Could you check a few things on this drawing? It's one solid part, dimensions in mm from its lowest x, y, z. A direction names the side the tool comes from. Give positions to 0.01 mm unless a question says otherwise; leave off trailing zeros. Write each loop counter-clockwise with the first axis right and the second up, starting at its lowest first coordinate (ties: lowest second). Pieces come first, ordered by that corner, then holes. Notation, with made-up numbers: (35, -30) -> (51, -30) arc R31 cw to (51, 3) -> close; hole circle Ø6 at (87.5, 31). An arc over 180 degrees is marked (long way). Answer as CSV lines item,"result". Start each with the question number.
1. If we section it at A-A on y = 29: Write out the boundary of the cut face in (x, z), plus the area to 3 significant figures.
2. I'm going to push flat-ended pins straight in: P1, Ø1.3, axis at x = 79.75, y = 37.35, coming from the +Z side; P2, Ø1, axis at x = 55, z = 6.5, coming from the +Y side. Where does each tip first touch, or does it pass through?
3. On a 3-axis mill with a long thin cutter (end or side, diameter ignored), from which of +Z, -Z, +X, -X, +Y, -Y can I reach the whole of each face in a straight line? I mean the marked faces 4 and 5. Say none if no direction works.
4. I need wall thicknesses on line 1 (Y direction, x = 60.5, z = 3); line 2 (Y direction, x = 45, z = 6.5); line 3 (Z direction, x = 79.5, y = 23.3). Which ranges of each line are inside material? Lowest first, please. Write a range as [from, to].
5. If we mould it in two halves opening along Y, with no side actions, what happens to the marked faces 1, 2 and 3? For each: pulls with the +Y half, pulls with the -Y half, needs draft (parallel to the pull), parting line crosses it, or undercut.
6. If we section it at C-C on y = 23.3: Write out the boundary of the cut face in (x, z), plus the area to 3 significant figures.
7. If we section it at D-D on x = 12.5: Write out the boundary of the cut face in (y, z).
8. If we section it at B-B on x = 79.75: Write out the boundary of the cut face in (y, z), plus the area to 3 significant figures.
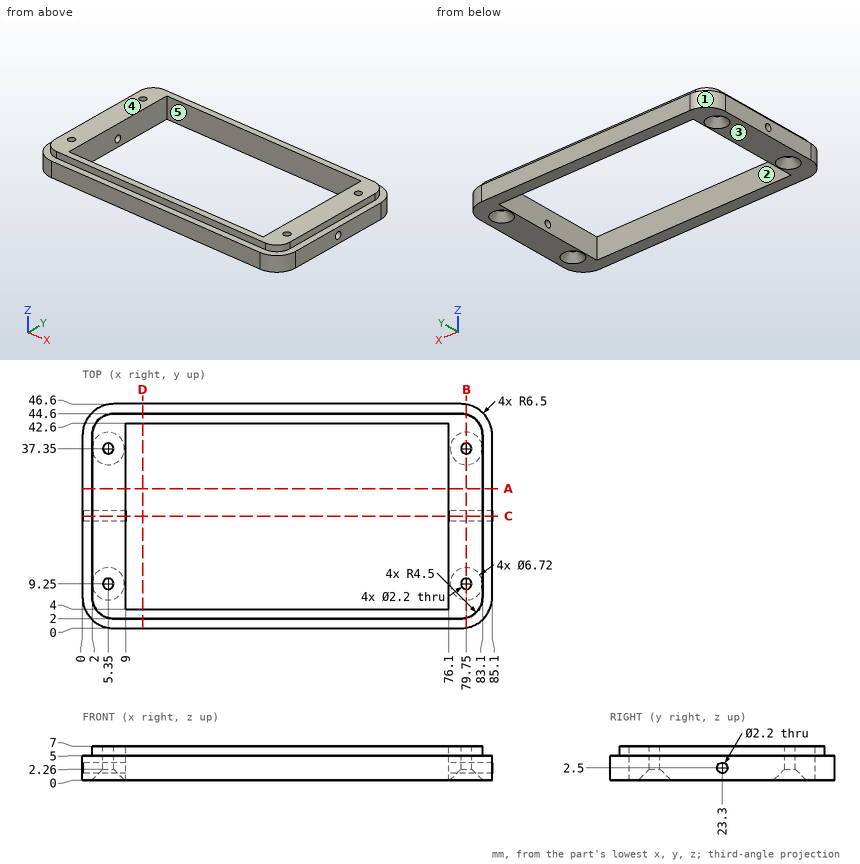
Computed values:
1,outline,"(0, 0) -> (9, 0) -> (9, 7) -> (2, 7) -> (2, 5) -> (0, 5) -> close; (76.1, 0) -> (85.1, 0) -> (85.1, 5) -> (83.1, 5) -> (83.1, 7) -> (76.1, 7) -> close"
1,area,"118 mm2"
2,P1,"passes through"
2,P2,"stops at y = 44.6"
3,face 4,"+Z, +X, -X, +Y, -Y"
3,face 5,"+Z, -Z"
4,line 1,"y = [0, 4], [42.6, 46.6]"
4,line 2,"y = [2, 4], [42.6, 44.6]"
4,line 3,"z = [0, 1.4], [3.6, 7]"
5,face 1,"pulls with the +Y half"
5,face 2,"undercut"
5,face 3,"needs draft"
6,outline,"(0, 0) -> (9, 0) -> (9, 1.4) -> (0, 1.4) -> close; (0, 3.6) -> (9, 3.6) -> (9, 7) -> (2, 7) -> (2, 5) -> (0, 5) -> close; (76.1, 0) -> (85.1, 0) -> (85.1, 1.4) -> (76.1, 1.4) -> close; (76.1, 3.6) -> (85.1, 3.6) -> (85.1, 5) -> (83.1, 5) -> (83.1, 7) -> (76.1, 7) -> close"
6,area,"78.4 mm2"
7,outline,"(0, 0) -> (4, 0) -> (4, 7) -> (2, 7) -> (2, 5) -> (0, 5) -> close; (42.6, 0) -> (46.6, 0) -> (46.6, 5) -> (44.6, 5) -> (44.6, 7) -> (42.6, 7) -> close"
8,outline,"(0.1, 0) -> (5.89, 0) -> (8.15, 2.26) -> (8.15, 7) -> (2.15, 7) -> (2.15, 5) -> (0.1, 5) -> close; (10.35, 2.26) -> (12.61, 0) -> (33.99, 0) -> (36.25, 2.26) -> (36.25, 7) -> (10.35, 7) -> close; (38.45, 2.26) -> (40.71, 0) -> (46.5, 0) -> (46.5, 5) -> (44.45, 5) -> (44.45, 7) -> (38.45, 7) -> close; hole circle Ø2.2 at (23.3, 2.5)"
8,area,"272 mm2"
